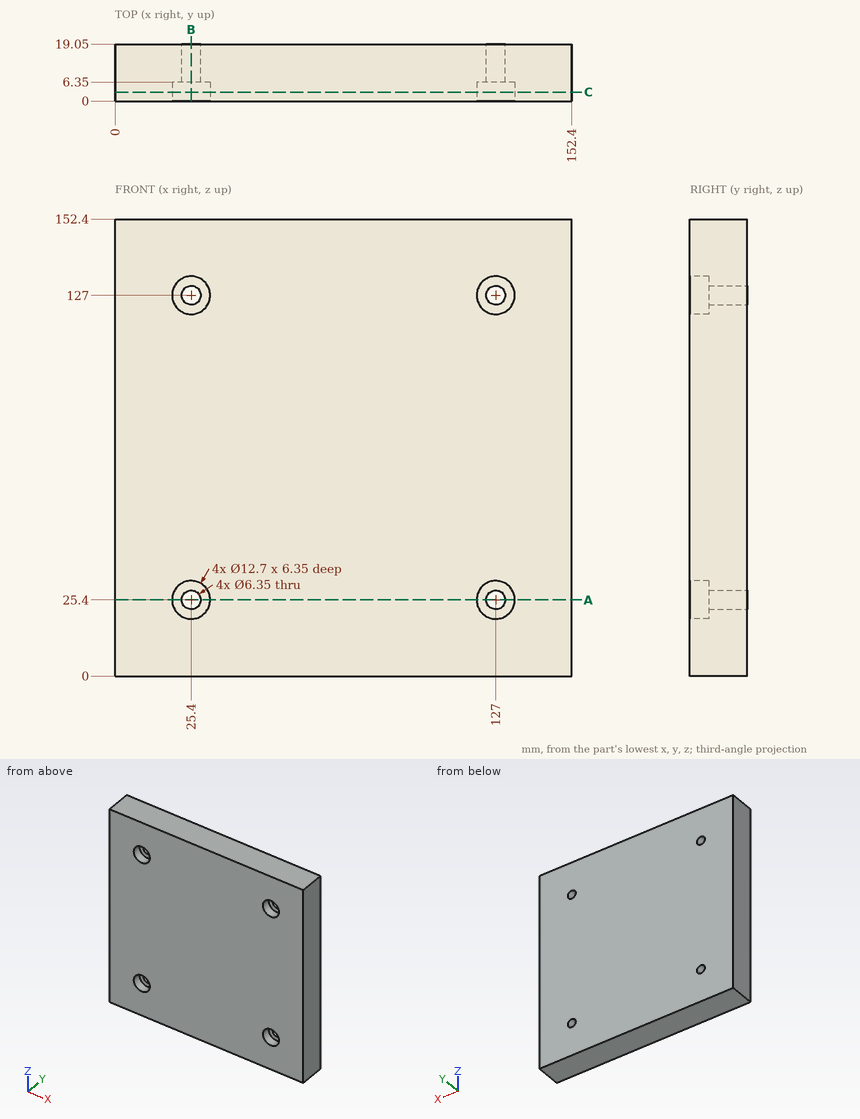
Design review of the part shown in the three views and the two pictorial views. Dimensions are in mm from the part's minimum x, y and z. Coordinates: 2 decimals unless noted, no trailing zeros. Loops run counter-clockwise (first coordinate to the right, second up) from the corner with the lowest first, then second, coordinate; pieces in that order, holes last.
(1) Consider section C-C, the plane y = 3. Give the boundary of the cut face in (x, z).
Determined:
outline: (0, 0) - (152.4, 0) - (152.4, 152.4) - (0, 152.4) - close; hole circle Ø12.7 at (25.4, 25.4); hole circle Ø12.7 at (25.4, 127); hole circle Ø12.7 at (127, 25.4); hole circle Ø12.7 at (127, 127)
(2) Insertion check: P1, Ø4, axis at x = 125.5, z = 127.5, coming from the -Y side. The pin has a flat end and moves straight along its axis. Give the tip position at first contact, or say it passes through.
Determined:
P1: stops at y = 6.35
(3) Consider section A-A, the plane z = 25.4. Give the boundary of the cut face in (x, y) (3 decimals), plus the area to 3 significant figures.
Determined:
outline: (0, 0) - (19.05, 0) - (19.05, 6.35) - (22.225, 6.35) - (22.225, 19.05) - (0, 19.05) - close; (28.575, 6.35) - (31.75, 6.35) - (31.75, 0) - (120.65, 0) - (120.65, 6.35) - (123.825, 6.35) - (123.825, 19.05) - (28.575, 19.05) - close; (130.175, 6.35) - (133.35, 6.35) - (133.35, 0) - (152.4, 0) - (152.4, 19.05) - (130.175, 19.05) - close
area: 2,580 mm2
(4) Wall thickness on L1, parallel to Z at x = 127, y = 11 (3 decimals); L2, parallel to Z at x = 127, y = 3: over which ranges is each line inside the solid? List them lowest first.
Determined:
L1: z = 0 to 22.225, 28.575 to 123.825, 130.175 to 152.4
L2: z = 0 to 19.05, 31.75 to 120.65, 133.35 to 152.4
(5) Consider section B-B, the plane x = 25.4. Give the boundary of the cut face in (y, z) (3 decimals).
Determined:
outline: (0, 0) - (19.05, 0) - (19.05, 22.225) - (6.35, 22.225) - (6.35, 19.05) - (0, 19.05) - close; (0, 31.75) - (6.35, 31.75) - (6.35, 28.575) - (19.05, 28.575) - (19.05, 123.825) - (6.35, 123.825) - (6.35, 120.65) - (0, 120.65) - close; (0, 133.35) - (6.35, 133.35) - (6.35, 130.175) - (19.05, 130.175) - (19.05, 152.4) - (0, 152.4) - close
